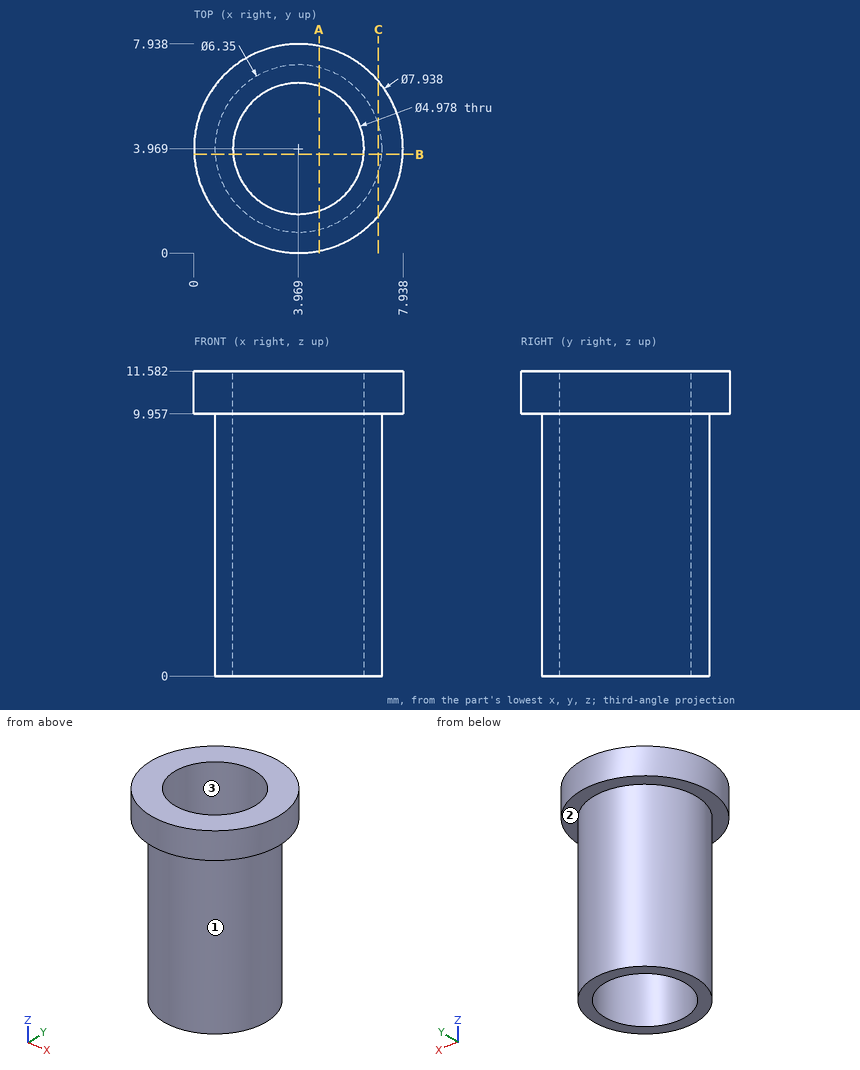
Verification items for this drawing (mm, ordinates from the low corner). Coordinates: 2 decimals unless noted, no trailing zeros. Loops run counter-clockwise (first coordinate to the right, second up) from the corner with the lowest first, then second, coordinate; pieces in that order, holes last.
Item 1: Thickness scan on line 1 (Y direction, x = 4, z = 1.5); line 2 (Z direction, x = 0.75, y = 2.5). Record the ranges inside material, lowest first.
Item 2: Sectioned sample at A-A, the plane x = 4.75. Record the boundary of the cut face in (y, z) (1 decimal).
Item 3: Go/stop test with flat-tipped pins: pin 1 Ø2 at (y, z) = (2.5, 2) entering from -X; pin 2 Ø1 at (x, z) = (4, 4) entering from -Y. Record where each tip stops, or that it passes through.
Item 4: Sectioned sample at C-C, the plane x = 7. Record the boundary of the cut face in (y, z).
Item 5: Release check for a two-part mould opening along Y. For the marked faces 1, 2 and 3 record: released by +Y, released by -Y, zero draft, split by the parting line, or undercut.
Item 6: Sectioned sample at B-B, the plane y = 3.75. Record the boundary of the cut face in (x, z).
Check result:
1. line 1: y = 0.79 to 1.48, 6.46 to 7.14
1. line 2: z = 9.96 to 11.58
2. outline: (0.1, 10) - (0.9, 10) - (0.9, 0) - (1.6, 0) - (1.6, 11.6) - (0.1, 11.6) - close; (6.3, 0) - (7, 0) - (7, 10) - (7.9, 10) - (7.9, 11.6) - (6.3, 11.6) - close
3. pin 1: stops at x = 0.83
3. pin 2: stops at y = 0.79
4. outline: (1.41, 9.96) - (3.02, 9.96) - (3.02, 0) - (4.91, 0) - (4.91, 9.96) - (6.53, 9.96) - (6.53, 11.58) - (1.41, 11.58) - close
5. face 1: split by the parting line
5. face 2: zero draft
5. face 3: undercut
6. outline: (0.01, 9.96) - (0.8, 9.96) - (0.8, 0) - (1.49, 0) - (1.49, 11.58) - (0.01, 11.58) - close; (6.45, 0) - (7.14, 0) - (7.14, 9.96) - (7.93, 9.96) - (7.93, 11.58) - (6.45, 11.58) - close
